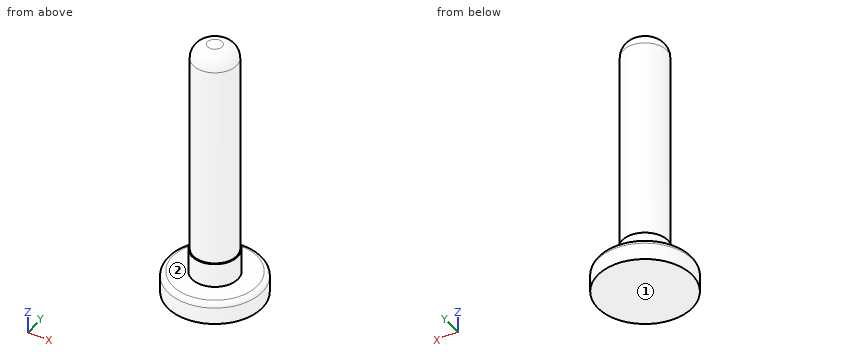
```python
from build123d import *

# Parameters (mm, degrees)
SKETCH1_R           = 9.75
BOSS_EXTRUDE1_DEPTH = 4.5
SKETCH2_R           = 4.75
BOSS_EXTRUDE2_DEPTH = 5
SKETCH3_R           = 4.5
BOSS_EXTRUDE3_DEPTH = 45
FILLET3_R           = 3
FILLET4_R           = 1


with BuildPart() as part:
    # Sketch1 → Boss-Extrude1 (new body)
    with BuildSketch(Plane.XY):
        Circle(SKETCH1_R)
    extrude(amount=BOSS_EXTRUDE1_DEPTH)

    # Sketch2 → Boss-Extrude2 (add)
    with BuildSketch(Plane.XY.offset(4.5)):
        Circle(SKETCH2_R)
    extrude(amount=BOSS_EXTRUDE2_DEPTH)

    # Sketch3 → Boss-Extrude3 (add)
    with BuildSketch(Plane.XY.offset(9.5)):
        with Locations(Location((0, 0, 0), (0, 0, 180))):
            Circle(SKETCH3_R)
    extrude(amount=BOSS_EXTRUDE3_DEPTH)

    # Fillet3
    fillet3_edges = [part.edges().sort_by_distance(p)[0] for p in [
        (4.5, 0, 54.5),
    ]]
    fillet(fillet3_edges, radius=FILLET3_R)

    # Fillet4
    fillet4_edges = [part.edges().sort_by_distance(p)[0] for p in [
        (-9.75, 0, 4.5),
    ]]
    fillet(fillet4_edges, radius=FILLET4_R)


solid = part.part
```
Geometry: final body of the model. Coordinates: model frame, mm. Face numbers are marked on the shaded views. A direction names the side the tool comes from. Coordinates: 2 decimals unless noted, no trailing zeros. Write each loop counter-clockwise with the first axis right and the second up, starting at its lowest first coordinate (ties: lowest second). Pieces come first, ordered by that corner, then holes. Notation, with made-up numbers: M 58,-16.5 L 86,-16.5 A25 ccw 86,8.5 Z; hole C 84.25,38 d11. An arc over 180 degrees is marked long. Use CSV: the item, a comma, the result in double quotes. Start each with the question number.
1. Reachability of the marked faces 1 and 2 from +Z, -Z, +X, -X, +Y, -Y: full face, straight path, thin tool, end or side. Return the list, or none.
2. First-contact query: P1, Ø4, axis at x = 4.5, z = 7, coming from the -Y side; P2, Ø6, axis at x = 1, z = 10, coming from the -Y side; P3, Ø6, axis at x = 4, z = 38.5, coming from the -Y side. Flat tips, straight axial feed; report the tip coordinate or a pass-through.
3. Ray query, probe 1 along Z at (x, y) = (-5, -4.75); probe 2 along X at (y, z) = (-0.25, 6); probe 3 along X at (y, z) = (-0.25, 16.5). Return the intervals inside material, ascending.
4. Cut plane A-A on z = 50. Return the cut outline in (x, y).
Entries:
1,face 1,"-Z, +X, -X, +Y, -Y"
1,face 2,"+Z"
2,P1,"y = -4.04"
2,P2,"y = -4.75"
2,P3,"y = -4.39"
3,probe 1,"0 to 4.5"
3,probe 2,"-4.74 to 4.74"
3,probe 3,"-4.49 to 4.49"
4,outline,"C 0,0 d9"
